Here's how the part is built. I have some questions about the finished solid (model axes, mm). Face numbers are marked on the shaded views. A direction names the side the tool comes from. Give positions to 0.01 mm unless a question says otherwise; leave off trailing zeros. Write each loop counter-clockwise with the first axis right and the second up, starting at its lowest first coordinate (ties: lowest second). Pieces come first, ordered by that corner, then holes. Notation, with made-up numbers: M -9,43 L 0,43 A20 cw 0,68 Z; hole C 48.25,84 d11. An arc over 180 degrees is marked long. Use one line per item in the form item = value. Start each with the question number.
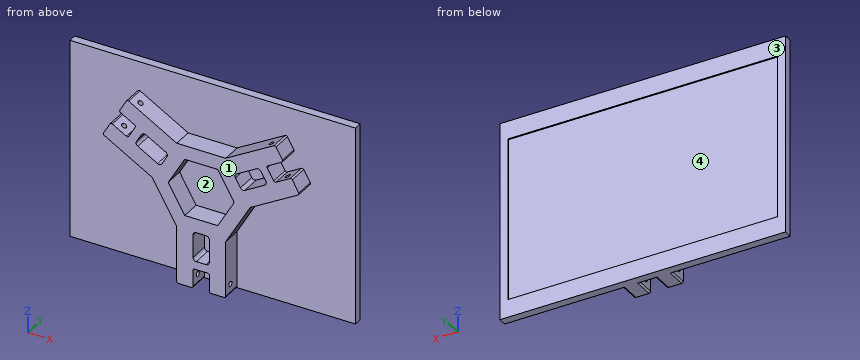
from build123d import *

# Parameters (mm, degrees)
CROQUIS1_W              = 10
CROQUIS1_H              = 18.019237886
SALIENTE_EXTRUIR1_DEPTH = 12
CORTAR_EXTRUIR1_REACH   = 99.669
CROQUIS2_R              = 1.55
CORTAR_EXTRUIR2_REACH   = 103.09
CROQUIS3_R              = 1.55
CORTAR_EXTRUIR3_REACH   = 91.077
CROQUIS4_R              = 1.55
CROQUIS6_W              = 175
CROQUIS6_H              = 122
SALIENTE_EXTRUIR7_DEPTH = 5
REDONDEO1_R             = 2
REDONDEO2_R             = 1
CROQUIS7_W              = 165
CROQUIS7_H              = 100
CORTAR_EXTRUIR4_DEPTH   = 0.8


with BuildPart() as part:
    # Croquis1 → Saliente-Extruir1 (new body)
    with BuildSketch(Plane(origin=(0, 0, 0), x_dir=(1, 0, 0), z_dir=(0, 1, 0))):
        Polygon((5, 49), (-5, 49), (-5, 61), (-15, 61), (-15, 25.980762114), (-30, 0), (-60.327549631, -17.509618943), (-55.327549631, -26.169872981), (-44.935244785, -20.169872981), (-39.935244785, -28.830127019), (-50.327549631, -34.830127019), (-45.327549631, -43.490381057), (-15, -25.980762114), (15, -25.980762114), (45.327549631, -43.490381057), (50.327549631, -34.830127019), (39.935244785, -28.830127019), (44.935244785, -20.169872981), (55.327549631, -26.169872981), (60.327549631, -17.509618943), (30, 0), (15, 25.980762114), (15, 61), (5, 61), align=None)
        Polygon((-40.605117767, -17.669872981), (-25, -8.660254038), (-20, -17.320508076), (-35.605117767, -26.330127019), align=None, mode=Mode.SUBTRACT)
        Polygon((10.103629711, 17.5), (20.207259422, 0), (10.103629711, -17.5), (-10.103629711, -17.5), (-20.207259422, 0), (-10.103629711, 17.5), align=None, mode=Mode.SUBTRACT)
        Polygon((25, -8.660254038), (40.605117767, -17.669872981), (35.605117767, -26.330127019), (20, -17.320508076), align=None, mode=Mode.SUBTRACT)
        with Locations((0, 34.990381057)):
            Rectangle(CROQUIS1_W, CROQUIS1_H, mode=Mode.SUBTRACT)
    extrude(amount=SALIENTE_EXTRUIR1_DEPTH)

    # Cortar-Extruir1: up to this face of the body (flat: up to its plane)
    cortar_extruir1_end = Plane(part.part.faces().sort_by_distance((15, 6, -43.490381057))[0])
    # Croquis2 → Cortar-Extruir1 (cut, up to the picked face)
    with BuildSketch(Plane.ZY.offset(15), mode=Mode.PRIVATE) as cortar_extruir1_sk1:
        with Locations((-55, 5)):
            Circle(CROQUIS2_R)
    cortar_extruir1_tool1 = split(extrude(cortar_extruir1_sk1.sketch, amount=-CORTAR_EXTRUIR1_REACH, mode=Mode.PRIVATE), bisect_by=cortar_extruir1_end, keep=Keep.BOTH, mode=Mode.PRIVATE)
    add(cortar_extruir1_tool1.solids().sort_by(Axis((-15, 5, -55), (1, 0, 0)))[0], mode=Mode.SUBTRACT)

    # Cortar-Extruir2: up to this face of the body (flat: up to its plane)
    cortar_extruir2_end = Plane(part.part.faces().sort_by_distance((-45.163774815, 6, 8.754809472))[0])
    # Croquis3 → Cortar-Extruir2 (cut, up to the picked face)
    with BuildSketch(Plane(origin=(7.5, 0, 12.990381057), x_dir=(0.8660254037844382, 0, -0.5000000000000007), z_dir=(0.5000000000000008, 0, 0.8660254037844383)), mode=Mode.PRIVATE) as cortar_extruir2_sk1:
        with Locations((-55, 5)):
            Circle(CROQUIS3_R)
    cortar_extruir2_tool1 = split(extrude(cortar_extruir2_sk1.sketch, amount=-CORTAR_EXTRUIR2_REACH, mode=Mode.PRIVATE), bisect_by=cortar_extruir2_end, keep=Keep.BOTH, mode=Mode.PRIVATE)
    add(cortar_extruir2_tool1.solids().sort_by(Axis((-40.131397, 5, 40.490381), (-0.5000000000000008, 0, -0.8660254037844383)))[0], mode=Mode.SUBTRACT)

    # Cortar-Extruir3: up to this face of the body (flat: up to its plane)
    cortar_extruir3_end = Plane(part.part.faces().sort_by_distance((30.163774815, 6, 34.735571585))[0])
    # Croquis4 → Cortar-Extruir3 (cut, up to the picked face)
    with BuildSketch(Plane(origin=(7.5, 0, -12.990381057), x_dir=(-0.8660254037844407, 0, -0.4999999999999965), z_dir=(0.49999999999999656, 0, -0.8660254037844407)), mode=Mode.PRIVATE) as cortar_extruir3_sk1:
        with Locations((-55, 5)):
            Circle(CROQUIS4_R)
    cortar_extruir3_tool1 = split(extrude(cortar_extruir3_sk1.sketch, amount=-CORTAR_EXTRUIR3_REACH, mode=Mode.PRIVATE), bisect_by=cortar_extruir3_end, keep=Keep.BOTH, mode=Mode.PRIVATE)
    add(cortar_extruir3_tool1.solids().sort_by(Axis((55.131397, 5, 14.509619), (-0.49999999999999656, 0, 0.8660254037844407)))[0], mode=Mode.SUBTRACT)

    # Croquis6 → Saliente-Extruir7 (add)
    with BuildSketch(Plane(origin=(0, 12, 0), x_dir=(1, 0, 0), z_dir=(0, 1, 0))):
        Rectangle(CROQUIS6_W, CROQUIS6_H)
    extrude(amount=SALIENTE_EXTRUIR7_DEPTH)

    # Redondeo1
    redondeo1_edges = [part.edges().sort_by_distance(p)[0] for p in [
        (35.605117767, 6, 26.330127019),
        (40.605117767, 6, 17.669872981),
        (25, 6, 8.660254038),
        (20, 6, 17.320508076),
        (-35.605117767, 6, 26.330127019),
        (-20, 6, 17.320508076),
        (-25, 6, 8.660254038),
        (-40.605117767, 6, 17.669872981),
        (-5, 6, -25.980762114),
        (5, 6, -25.980762114),
        (5, 6, -44),
        (-5, 6, -44),
    ]]
    fillet(redondeo1_edges, radius=REDONDEO1_R)

    # Redondeo2
    redondeo2_edges = [part.edges().sort_by_distance(p)[0] for p in [
        (-15, 6, -61),
        (-5, 6, -61),
        (-5, 6, -49),
        (5, 6, -49),
        (5, 6, -61),
        (15, 6, -61),
        (60.327549631, 6, 17.509618943),
        (55.327549631, 6, 26.169872981),
        (44.935244785, 6, 20.169872981),
        (39.935244785, 6, 28.830127019),
        (50.327549631, 6, 34.830127019),
        (45.327549631, 6, 43.490381057),
        (-45.327549631, 6, 43.490381057),
        (-50.327549631, 6, 34.830127019),
        (-39.935244785, 6, 28.830127019),
        (-44.935244785, 6, 20.169872981),
        (-55.327549631, 6, 26.169872981),
        (-60.327549631, 6, 17.509618943),
    ]]
    fillet(redondeo2_edges, radius=REDONDEO2_R)

    # Croquis7 → Cortar-Extruir4 (cut)
    with BuildSketch(Plane(origin=(0, 17, 0), x_dir=(1, 0, 0), z_dir=(0, 1, 0))):
        Rectangle(CROQUIS7_W, CROQUIS7_H)
    extrude(amount=-CORTAR_EXTRUIR4_DEPTH, mode=Mode.SUBTRACT)


solid = part.part
1) Suppose I cut it at B-B, the plane z = -8. List the corners of the cut face in (x, y) for me, and give its area (3 significant figures).
2) Suppose I cut it at D-D, the plane z = 4.5. List the corners of the cut face in (x, y) for me.
3) On a 3-axis mill with a long thin cutter (end or side, diameter ignored), from which of +Z, -Z, +X, -X, +Y, -Y can I reach the whole of each face in a straight line? I mean the marked faces 1 and 2. Say none if no direction works.
4) Suppose I cut it at A-A, the plane x = 62. List the corners of the cut face in (y, z) for me.
5) Suppose I cut it at C-C, the plane x = 12. List the corners of the cut face in (y, z) for me, and give its area (3 significant figures).
6) Please list where these lines run through material, in increasing order: line 1 (Y direction, x = 12.25, z = -55); line 2 (X direction, y = 2.5, z = -50.5); line 3 (Y direction, x = 62, z = 41).
7) Will these pins go through, and if not, where does the flat tip stop? P1, Ø5, axis at x = 29, z = 19.5, coming from the -Y side; P2, Ø9.5, axis at x = 0.5, y = 3.5, coming from the -Z side; P3, Ø6, axis at y = 4.5, z = -35.5, coming from the +X side.
8) Thinking about a two-plate mould opening in X: for the marked faces 3 and 4, which applies, released by +X, released by -X, zero draft, split by the parting line, or undercut?
Checks:
q1.outline = M -87.5,12 L -25.38,12 L -25.38,0 L -15.59,0 L -15.59,12 L 15.59,12 L 15.59,0 L 25.38,0 L 25.38,12 L 87.5,12 L 87.5,17 L 82.5,17 L 82.5,16.2 L -82.5,16.2 L -82.5,17 L -87.5,17 Z
q1.area = 978 mm^2
q2.outline = M -87.5,12 L -37.79,12 L -37.79,0 L -17.61,0 L -17.61,12 L 17.61,12 L 17.61,0 L 37.79,0 L 37.79,12 L 87.5,12 L 87.5,17 L 82.5,17 L 82.5,16.2 L -82.5,16.2 L -82.5,17 L -87.5,17 Z
q3.face_1 = +Z, -Z, +X, -X, -Y
q3.face_2 = -Y
q4.outline = M 12,-61 L 17,-61 L 17,-50 L 16.2,-50 L 16.2,50 L 17,50 L 17,61 L 12,61 Z
q5.outline = M 0,-61 L 17,-61 L 17,-50 L 16.2,-50 L 16.2,50 L 17,50 L 17,61 L 12,61 L 12,25.98 L 0,25.98 L 0,14.22 L 12,14.22 L 12,-14.22 L 0,-14.22 Z; hole C 5,-55 d3.1
q5.area = 1,230 mm^2
q6.line_1 = 0 to 3.45, 6.55 to 17
q6.line_2 = -15 to -5, 5 to 15
q6.line_3 = 12 to 16.2
q7.P1 = 12
q7.P2 = -60.66
q7.P3 = 15
q8.face_3 = zero draft
q8.face_4 = undercut
